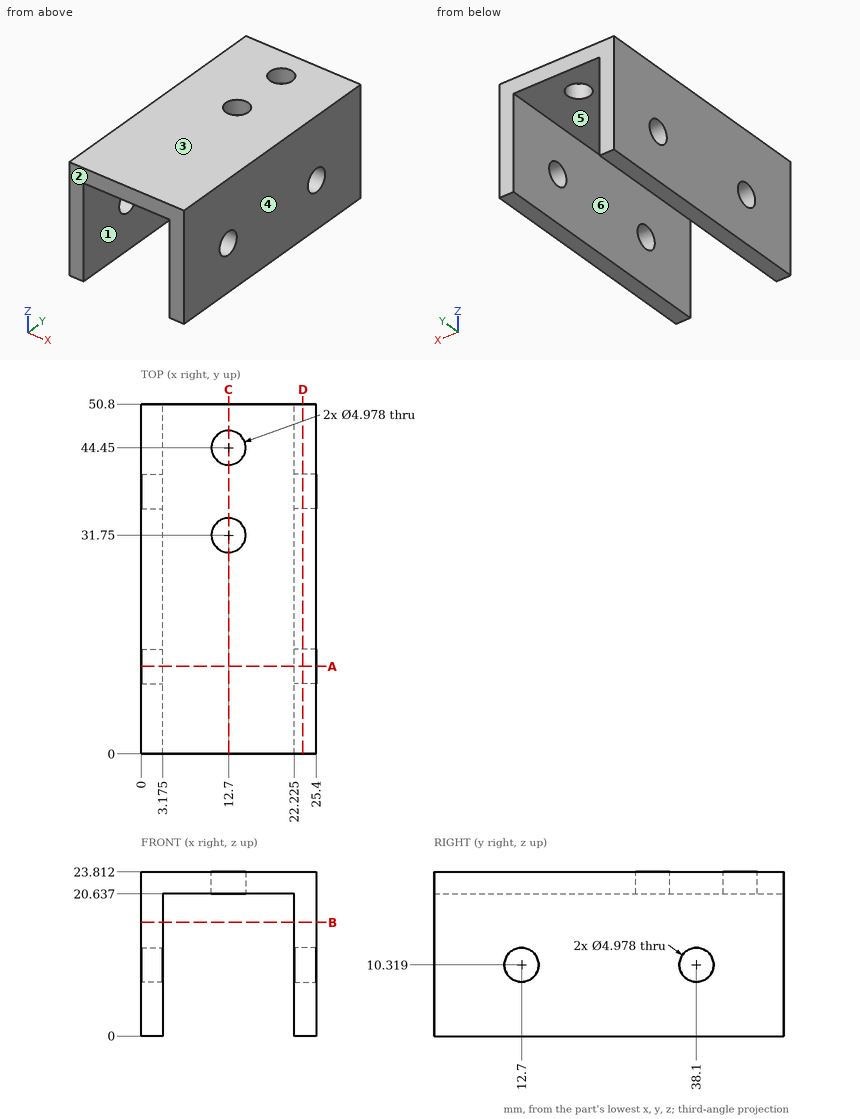
Could you check a few things on this drawing? It's one solid part, dimensions in mm from its lowest x, y, z. A direction names the side the tool comes from. Coordinates: 2 decimals unless noted, no trailing zeros. Loops run counter-clockwise (first coordinate to the right, second up) from the corner with the lowest first, then second, coordinate; pieces in that order, holes last.
1. Imagine slicing it at B-B (z = 16.5). Please give me the cut outline in (x, y) (1 decimal).
2. Imagine slicing it at A-A (y = 12.7). Please give me the cut outline in (x, z) (1 decimal).
3. We'd pull the mould along X, two halves only. Please class the marked faces 3, 4, 5 and 6: released by +X, released by -X, zero draft, split by the parting line, or undercut.
4. Imagine slicing it at D-D (x = 23.5). Please give me the cut outline in (y, z).
5. For P1, Ø6, axis at x = 19, y = 10.5, coming from the -Z side; P2, Ø1.5, axis at x = 18, z = 19, coming from the +Y side, each with a flat end and sliding along its axis, tell me the tip position at first contact or that it passes through.
6. For the marked faces 1 and 2, which set-ups out of +Z, -Z, +X, -X, +Y, -Y let a thin tool reach every point of the face, with its end or its side?
7. Imagine slicing it at C-C (x = 12.7). Please give me the cut outline in (y, z), and give its area (3 significant figures).
8. I need wall thicknesses on L1, parallel to Y at x = 12.7, z = 21.55; L2, parallel to X at y = 9.5, z = 5.25 (1 decimal); L3, parallel to Z at x = 12.25, y = 10. Which ranges of each line are inside material? Lowest first, please.
Computed values:
1. outline: (0, 0) - (3.2, 0) - (3.2, 50.8) - (0, 50.8) - close; (22.2, 0) - (25.4, 0) - (25.4, 50.8) - (22.2, 50.8) - close
2. outline: (0, 0) - (3.2, 0) - (3.2, 7.8) - (0, 7.8) - close; (0, 12.8) - (3.2, 12.8) - (3.2, 20.6) - (22.2, 20.6) - (22.2, 12.8) - (25.4, 12.8) - (25.4, 23.8) - (0, 23.8) - close; (22.2, 0) - (25.4, 0) - (25.4, 7.8) - (22.2, 7.8) - close
3. face 3: zero draft
3. face 4: released by +X
3. face 5: undercut
3. face 6: undercut
4. outline: (0, 0) - (50.8, 0) - (50.8, 23.81) - (0, 23.81) - close; hole circle Ø4.98 at (12.7, 10.32); hole circle Ø4.98 at (38.1, 10.32)
5. P1: stops at z = 20.64
5. P2: passes through
6. face 1: -Z, +Y, -Y
6. face 2: +Z, -Z, +X, -X, -Y
7. outline: (0, 20.64) - (29.26, 20.64) - (29.26, 23.81) - (0, 23.81) - close; (34.24, 20.64) - (41.96, 20.64) - (41.96, 23.81) - (34.24, 23.81) - close; (46.94, 20.64) - (50.8, 20.64) - (50.8, 23.81) - (46.94, 23.81) - close
7. area: 130 mm2
8. L1: y = 0 to 29.26, 34.24 to 41.96, 46.94 to 50.8
8. L2: x = 0 to 3.2, 22.2 to 25.4
8. L3: z = 20.64 to 23.81
